from build123d import *

# Parameters (mm, degrees)
BOSS_EXTRU_1_DEPTH         = 215
ESQUISSE3_W                = 8
ESQUISSE3_H                = 7.5
ESQUISSE3_W_2              = 11
ENL_V_MAT_EXTRU_1_DEPTH    = 3
ESQUISSE4_W                = 11
ESQUISSE4_H                = 6
ENL_V_MAT_EXTRU_2_DEPTH    = 217.531752868
ESQUISSE5_W                = 6
ESQUISSE5_H                = 6
ENL_V_MAT_EXTRU_3_DEPTH    = 3
ESQUISSE8_R                = 2.5
ENL_V_MAT_EXTRU_4_DEPTH    = 10
R_P_TITION_LIN_AIRE1_COUNT = 2
R_P_TITION_LIN_AIRE1_PITCH = 9


with BuildPart() as part:
    # Esquisse1 → Boss.-Extru.1 (new body)
    with BuildSketch(Plane.XY):
        Polygon((0, 0), (0, 6), (20, 6), (20, 3), (25, 3), (25, 0), align=None)
    extrude(amount=BOSS_EXTRU_1_DEPTH)

    # Esquisse3 → Enlèv. mat.-Extru.1 (cut)
    with BuildSketch(Plane.XZ):
        with Locations((21, 174.174574215)):
            Rectangle(ESQUISSE3_W, ESQUISSE3_H)
        with Locations((5.5, 174.174574215)):
            Rectangle(ESQUISSE3_W_2, ESQUISSE3_H)
    extrude(amount=-ENL_V_MAT_EXTRU_1_DEPTH, mode=Mode.SUBTRACT)

    # Esquisse4 → Enlèv. mat.-Extru.2 (cut, through all)
    with BuildSketch(Plane.XZ):
        with Locations((5.5, 142)):
            Rectangle(ESQUISSE4_W, ESQUISSE4_H)
    extrude(amount=-ENL_V_MAT_EXTRU_2_DEPTH, mode=Mode.SUBTRACT)

    # Esquisse5 → Enlèv. mat.-Extru.3 (cut)
    with BuildSketch(Plane.XZ):
        with Locations((22, 142)):
            Rectangle(ESQUISSE5_W, ESQUISSE5_H)
    extrude(amount=-ENL_V_MAT_EXTRU_3_DEPTH, mode=Mode.SUBTRACT)

    # Esquisse8 → Enlèv. mat.-Extru.4 (cut)
    with BuildSketch(Plane.XY.offset(215)):
        with Locations((5, 3)):
            Circle(ESQUISSE8_R)
    enl_v_mat_extru_4 = extrude(amount=-ENL_V_MAT_EXTRU_4_DEPTH, mode=Mode.SUBTRACT)

    # Répétition linéaire1: Enlèv. mat.-Extru.4 ×2
    with Locations(*[(i * R_P_TITION_LIN_AIRE1_PITCH, 0, 0) for i in range(1, R_P_TITION_LIN_AIRE1_COUNT)]):
        add(enl_v_mat_extru_4, mode=Mode.SUBTRACT)


solid = part.part
Input: part model. Units: mm. Frame: model coordinates. A direction names the side the tool comes from. Coordinates: 2 decimals unless noted, no trailing zeros. Loops run counter-clockwise (first coordinate to the right, second up) from the corner with the lowest first, then second, coordinate; pieces in that order, holes last.
Q1. Cut plane B-B (x = 5). Output: boundary loops of the cut face in (y, z).
Q2. Contact query for flat-ended pins moving along their axis: pin 1 (2.5 mm diameter, centred on x = 6, y = 1.5, fed in from +Z); pin 2 (4 mm diameter, centred on x = 6, z = 173.5, fed in from -Y); pin 3 (1.5 mm diameter, centred on x = 22, z = 75, fed in from +Y); pin 4 (1.5 mm diameter, centred on y = 4.5, z = 96.5, fed in from +X). Output: stop coordinate, or through.
Q3. Set-up query: faces 5 (the face through (11, 3, 142)), 6 (the face through (22, 3, 158)), 7 (the face through (14, 3, 205)). Return all of +Z, -Z, +X, -X, +Y, -Y with unobstructed straight access to the full face (end or side cutting, diameter ignored); none if empty.
Q4. Cut plane C-C (z = 104.5). Output: boundary loops of the cut face in (x, y).
Q5. Material intervals for line 1 (Z direction, x = 21, y = 0.45); line 2 (Z direction, x = 5.5, y = 2.7); line 3 (Z direction, x = 18, y = 1.5), sorted ascending.
Q6. Draft query along Z for faces 1 (the face through (10, 3, 215)), 2 (the face through (5, 3, 174)), 3 (the face through (5, 3, 145)), 4 (the face through (22, 3, 196)). Return one class per face: +Z half, -Z half, draft (parallel to the pull), parting line (faces both ways), or undercut.
Q7. Cut plane D-D (y = 4.6). Output: boundary loops of the cut face in (x, z).
Q8. Cut plane A-A (x = 14). Output: boundary loops of the cut face in (y, z), then the cut area to 3 significant figures.
Working result:
1. outline: (0, 0) - (6, 0) - (6, 139) - (0, 139) - close; (0, 145) - (6, 145) - (6, 215) - (5.5, 215) - (5.5, 205) - (0.5, 205) - (0.5, 215) - (0, 215) - (0, 177.92) - (3, 177.92) - (3, 170.42) - (0, 170.42) - close
2. pin 1: stops at z = 215
2. pin 2: stops at y = 3
2. pin 3: stops at y = 3
2. pin 4: stops at x = 20
3. face 5: -X, +Y, -Y
3. face 6: +Z, -Z, +X, +Y
3. face 7: +Z
4. outline: (0, 0) - (25, 0) - (25, 3) - (20, 3) - (20, 6) - (0, 6) - close
5. line 1: z = 0 to 139, 145 to 170.42, 177.92 to 215
5. line 2: z = 0 to 139, 145 to 170.42, 177.92 to 205
5. line 3: z = 0 to 170.42, 177.92 to 215
6. face 1: +Z half
6. face 2: undercut
6. face 3: undercut
6. face 4: draft
7. outline: (0, 0) - (20, 0) - (20, 215) - (15.92, 215) - (15.92, 205) - (12.08, 205) - (12.08, 215) - (6.92, 215) - (6.92, 205) - (3.08, 205) - (3.08, 215) - (0, 215) - (0, 145) - (11, 145) - (11, 139) - (0, 139) - close
8. outline: (0, 0) - (6, 0) - (6, 215) - (5.5, 215) - (5.5, 205) - (0.5, 205) - (0.5, 215) - (0, 215) - close
8. area: 1,240 mm2
